Can you work these out from the model? Positions are in its coordinate system, mm. A direction names the side the tool comes from. Give positions to 0.01 mm unless a question says otherwise; leave off trailing zeros.
Item 1: Which directions (+Z, -Z, +X, -X, +Y, -Y) give clear straight access to the entire face, cutting with the end or side of a thin tool? Please do faces 1 (the cylindrical face through (29.43, -1.08, 3.42)), 2 (the cylindrical face through (-25.617, -1.092, 8.398)).
Item 2: If I drill on line 1 along X through (y, z) = (18, 5.25); line 2 along X through (y, z) = (-24.5, 6.5); line 3 along Y through (x, z) = (-13, 2), over which ranges is the centre line in solid material (lowest first)?
Item 3: I want a section at A-A, the plane z = 3.25. Count the separate pieces of the cut face and the enclosed holes in it, then the cut area to 3 significant figures.
Item 4: If we mould it in two halves opening along Y, with no side actions, what happens to faces 3 (the cylindrical face through (-16.328, -15.946, 5.07)), 4 (the cylindrical face through (13.778, -26.027, 3.422))? For each: +Y half, -Y half, draft (parallel to the pull), parting line (faces both ways), or undercut.
Item 5: I'm going to push flat-ended pins straight in: pin 1 Ø3 at (y, z) = (4, 4) entering from -X; pin 2 Ø5 at (x, z) = (12.5, 7) entering from +Y; pin 3 Ø10 at (x, y) = (0, 19.5) entering from -Z; pin 4 Ø1.9 at (x, y) = (14.13, 24.47) entering from -Z. Where does each tip first touch, or does it pass through?
```python
from build123d import *

# Parameters (mm, degrees)
SKETCH003_R           = 33
PAD_DEPTH             = 10
CHAMFER_SIZE          = 1.5
SKETCH_R              = 1.6
POCKET_DEPTH          = 197.745507
POLARPATTERN_COUNT    = 6
SKETCH001_R           = 2.85
POCKET001_DEPTH       = 3.25
POLARPATTERN001_COUNT = 6
SKETCH002_R           = 1.25
POCKET002_DEPTH       = 10.001
SKETCH004_R           = 1.25
POCKET003_DEPTH       = 10.001


with BuildPart() as part:
    # Sketch003 → Pad (new body)
    with BuildSketch(Plane.XY):
        Circle(SKETCH003_R)
    extrude(amount=PAD_DEPTH)

    # Chamfer
    chamfer_edges = [part.edges().sort_by_distance(p)[0] for p in [
        (-33, 0, 0),
    ]]
    chamfer(chamfer_edges, length=CHAMFER_SIZE)

    # Sketch → Pocket (cut, through all)
    with BuildSketch(Plane.XY.offset(10)):
        with Locations((-28.25, 0)):
            Circle(SKETCH_R)
    pocket = extrude(amount=-POCKET_DEPTH, mode=Mode.SUBTRACT)

    # PolarPattern: Pocket ×6 about axis
    polarpattern_axis = Axis((0, 0, 10), (0, 0, 1))
    for i in range(1, POLARPATTERN_COUNT):
        add(pocket.rotate(polarpattern_axis, i * 360 / POLARPATTERN_COUNT), mode=Mode.SUBTRACT)

    # Sketch001 → Pocket001 (cut)
    with BuildSketch(Plane.XY.offset(10)):
        with Locations((14.125, 24.465218)):
            Circle(SKETCH001_R)
    pocket001 = extrude(amount=-POCKET001_DEPTH, mode=Mode.SUBTRACT)

    # PolarPattern001: Pocket001 ×6 about axis
    polarpattern001_axis = Axis((0, 0, 10), (0, 0, 1))
    for i in range(1, POLARPATTERN001_COUNT):
        add(pocket001.rotate(polarpattern001_axis, i * 360 / POLARPATTERN001_COUNT), mode=Mode.SUBTRACT)

    # Sketch002 → Pocket002 (cut, through all)
    with BuildSketch(Plane.XY.offset(10)):
        with Locations((-17, 17)):
            Circle(SKETCH002_R)
        with Locations((17, 17)):
            Circle(SKETCH002_R)
        with Locations((-17, -17)):
            Circle(SKETCH002_R)
        with Locations((17, -17)):
            Circle(SKETCH002_R)
    extrude(amount=-POCKET002_DEPTH, mode=Mode.SUBTRACT)

    # Sketch004 → Pocket003 (cut, through all)
    with BuildSketch(Plane.XY.offset(10)):
        with Locations((-21.75, 0)):
            Circle(SKETCH004_R)
        with Locations((21.75, 0)):
            Circle(SKETCH004_R)
    extrude(amount=-POCKET003_DEPTH, mode=Mode.SUBTRACT)


solid = part.part
```
Results list:
1. face 1: +Z, -Z
1. face 2: +Z
2. line 1: x = -27.66 to -17.75, -16.25 to 16.25, 17.75 to 27.66
2. line 2: x = -22.11 to -15.72, -12.53 to 12.53, 15.72 to 22.11
2. line 3: y = -30.33 to -25.6, -23.33 to 23.33, 25.6 to 30.33
3. separate pieces: 1
3. enclosed holes: 12
3. area: 3,340 mm2
4. face 3: undercut
4. face 4: undercut
5. pin 1: stops at x = -32.91
5. pin 2: stops at y = 31.45
5. pin 3: stops at z = 0
5. pin 4: passes through
